Could you check a few things on this drawing? It's one solid part, dimensions in mm from its lowest x, y, z. Round coordinates to 2 decimals unless told otherwise and drop trailing zeros. Write each loop counter-clockwise with the first axis right and the second up, starting at its lowest first coordinate (ties: lowest second). Pieces come first, ordered by that corner, then holes. Notation, with made-up numbers: (28.5, 20.5) - (44.5, 20.5) arc R10 cw to (44.5, 27.5) - close; hole circle Ø6 at (45, -10). An arc over 180 degrees is marked (long way). Put each result on its own line as item: value.
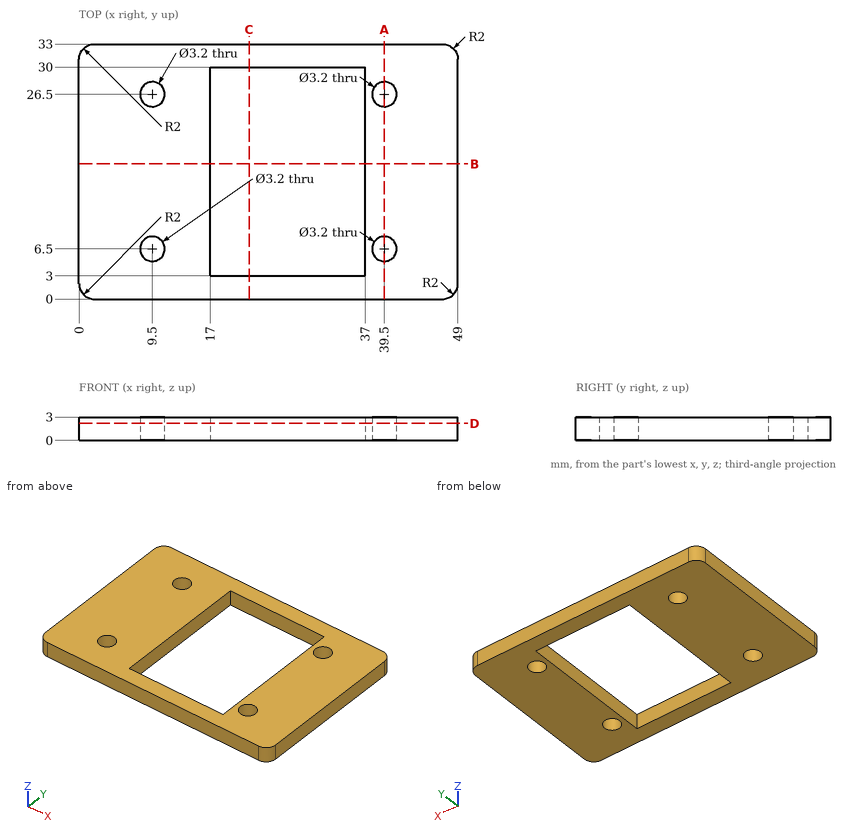
(1) Imagine slicing it at D-D, the plane z = 2.2. List the corners of the cut face in (x, y) for me, then the cut area to 3 significant figures.
Values found:
outline: (0, 2) arc R2 ccw to (2, 0) - (47, 0) arc R2 ccw to (49, 2) - (49, 31) arc R2 ccw to (47, 33) - (2, 33) arc R2 ccw to (0, 31) - close; hole circle Ø3.2 at (9.5, 6.5); hole circle Ø3.2 at (9.5, 26.5); hole (17, 3) - (37, 3) - (37, 30) - (17, 30) - close; hole circle Ø3.2 at (39.5, 6.5); hole circle Ø3.2 at (39.5, 26.5)
area: 1,040 mm^2
(2) Imagine slicing it at B-B, the plane y = 17.5. List the corners of the cut face in (x, z) for me, then the cut area to 3 significant figures.
Values found:
outline: (0, 0) - (17, 0) - (17, 3) - (0, 3) - close; (37, 0) - (49, 0) - (49, 3) - (37, 3) - close
area: 87.0 mm^2
(3) Please list where these lines run through material, in increasing order: probe 1 along Y at (x, z) = (39.5, 1.4); probe 2 along X at (y, z) = (14, 0.7); probe 3 along Y at (x, z) = (36, 2.8). Write a range as from..to.
Values found:
probe 1: y = 0..4.9, 8.1..24.9, 28.1..33
probe 2: x = 0..17, 37..49
probe 3: y = 0..3, 30..33
(4) Imagine slicing it at C-C, the plane x = 22. List the corners of the cut face in (y, z) for me.
Values found:
outline: (0, 0) - (3, 0) - (3, 3) - (0, 3) - close; (30, 0) - (33, 0) - (33, 3) - (30, 3) - close
(5) Imagine slicing it at A-A, the plane x = 39.5. List the corners of the cut face in (y, z) for me.
Values found:
outline: (0, 0) - (4.9, 0) - (4.9, 3) - (0, 3) - close; (8.1, 0) - (24.9, 0) - (24.9, 3) - (8.1, 3) - close; (28.1, 0) - (33, 0) - (33, 3) - (28.1, 3) - close
